Can you work these out from the model? Positions are in its coordinate system, mm. Round coordinates to 2 decimals unless told otherwise and drop trailing zeros. Loops run counter-clockwise (first coordinate to the right, second up) from the corner with the lowest first, then second, coordinate; pieces in that order, holes last. Notation, with made-up numbers: (37, 85) -> (79, 85) arc R6 ccw to (79, 93) -> close; hole circle Ø5 at (28, 77.5). An arc over 180 degrees is marked (long way). Write each question's results on one line, items separated by ' | '.
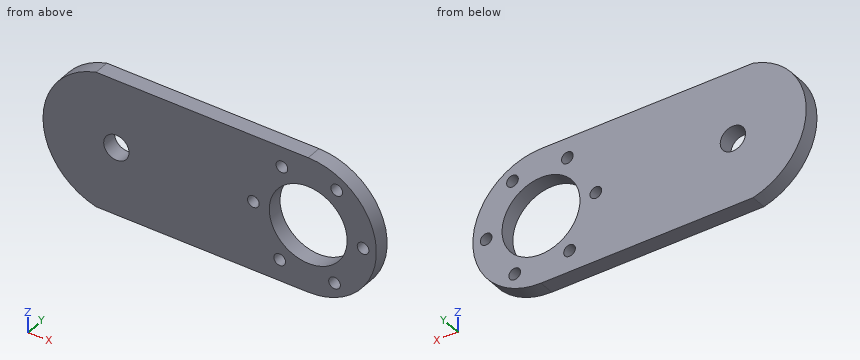
from build123d import *

# Parameters (mm, degrees)
SKETCH_1_R          = 6.5
SKETCH_1_R_2        = 20
EXTRUDE_1_DEPTH     = 8
SKETCH_2_R          = 3
CUT_EXTRUDE_1_DEPTH = 10


with BuildPart() as part:
    # Эскиз1 → Вытянуть1 (new body)
    with BuildSketch(Plane(origin=(0, 0, 0), x_dir=(1, 0, 0), z_dir=(0, 1, 0))):
        with BuildLine():
            Line((1.738556374, 18.516613497), (110.672099026, 18.516613497))
            ThreePointArc((110.672099026, 18.516613497), (145.672099026, -16.483386503), (110.672099026, -51.483386503))
            Line((110.672099026, -51.483386503), (1.738556374, -51.483386503))
            ThreePointArc((1.738556374, -51.483386503), (-25.499232193, -16.483386503), (1.738556374, 18.516613497))
        make_face()
        with Locations(Location((12.165325646, -16.483386503, 0), (0, 0, 270))):
            Circle(SKETCH_1_R, mode=Mode.SUBTRACT)
        with Locations(Location((110.670387559, -16.483386503, 0), (0, 0, 270))):
            Circle(SKETCH_1_R_2, mode=Mode.SUBTRACT)
    extrude(amount=EXTRUDE_1_DEPTH)

    # Эскиз2 → Вырез-Вытянуть1 (cut)
    with BuildSketch(Plane(origin=(0, 8, 0), x_dir=(1, 0, 0), z_dir=(0, 1, 0))):
        with Locations(Location((96.021590781, 7.563843825, 0), (0, 0, 270))):
            Circle(SKETCH_2_R)
        with Locations(Location((124.179862127, 8.221889416, 0), (0, 0, 270))):
            Circle(SKETCH_2_R)
        with Locations(Location((138.828881998, -15.834866101, 0), (0, 0, 270))):
            Circle(SKETCH_2_R)
        with Locations(Location((125.319630524, -40.549667208, 0), (0, 0, 270))):
            Circle(SKETCH_2_R)
        with Locations(Location((97.161359178, -41.207712799, 0), (0, 0, 270))):
            Circle(SKETCH_2_R)
        with Locations(Location((82.512339307, -17.150957282, 0), (0, 0, 270))):
            Circle(SKETCH_2_R)
    extrude(amount=-CUT_EXTRUDE_1_DEPTH, mode=Mode.SUBTRACT)


solid = part.part
1. If we section it at B-B (y = 6): State how many separate pieces and enclosed holes the cut face has, then the cut area to 3 significant figures.
Final values:
separate pieces: 1 | enclosed holes: 8 | area: 9,400 mm2
2. If we section it at C-C (x = 133): List the corners of the cut face in (y, z) for me, then the cut area to 3 significant figures.
Final values:
outline: (0, -10.47) -> (8, -10.47) -> (8, 43.44) -> (0, 43.44) -> close | area: 431 mm2
3. If we section it at A-A (z = 42): List the corners of the cut face in (x, y) for me, then the cut area to 3 significant figures.
Final values:
outline: (-14.94, 0) -> (94.27, 0) -> (94.27, 8) -> (-14.94, 8) -> close; (100.05, 0) -> (122.69, 0) -> (122.69, 8) -> (100.05, 8) -> close; (127.95, 0) -> (134.63, 0) -> (134.63, 8) -> (127.95, 8) -> close | area: 1,110 mm2
4. Will this pin go through, and if not, where does the flat tip stop? pin 1 (1.5 mm diameter, centred on y = 3, z = 19, fed in from -X).
Final values:
pin 1: x = -25.46
5. Please list where these lines run through material, in increasing order: line 1 (X direction, y = 4.75, z = -8.5); line 2 (Z direction, x = 96, y = 7.75); line 3 (X direction, y = 7.75, z = 21). Write a range as from..to.
Final values:
line 1: -15.46..93.17, 98.87..121.19, 127.17..135.18 | line 2: -18.52..-10.56, -4.56..2.89, 30.08..38.44, 43.97..51.48 | line 3: -25.22..7.49, 16.84..91.19, 130.15..145.38
